from build123d import *

# Parameters (mm, degrees)
F0_W     = 1054.1
F0_H     = 781.05
F1_DEPTH = 304.8
F0_R     = 25.4
F2_DEPTH = 25.4
F3_R     = 12.7
F4_SIZE  = 3.175
F5_R     = 12.7


with BuildPart() as f1:
    # F0 (on Top) → F1 (new body)
    with BuildSketch(Plane.XY):
        Rectangle(F0_W, F0_H)
        with BuildLine():
            ThreePointArc((-24.260394, 317.953571), (-15.749117, 333.525595), (0.879086, 339.725))
            Line((0.879086, 339.725), (450.85, 339.725))
            ThreePointArc((450.85, 339.725), (468.810512, 332.285512), (476.25, 314.325))
            Line((476.25, 314.325), (476.25, -314.325))
            ThreePointArc((476.25, -314.325), (468.810512, -332.285512), (450.85, -339.725))
            Line((450.85, -339.725), (-450.85, -339.725))
            ThreePointArc((-450.85, -339.725), (-468.810512, -332.285512), (-476.25, -314.325))
            Line((-476.25, -314.325), (-476.25, -137.404086))
            ThreePointArc((-476.25, -137.404086), (-470.050595, -120.775883), (-454.478571, -112.264606))
            ThreePointArc((-454.478571, -112.264606), (-167.839755, 31.314755), (-24.260394, 317.953571))
        make_face(mode=Mode.SUBTRACT)
    extrude(amount=F1_DEPTH)

    # F0 (on Top) → F2 (join)
    with BuildSketch(Plane.XY):
        with BuildLine():
            Line((450.85, 339.725), (0.879086, 339.725))
            ThreePointArc((0.879086, 339.725), (-15.749117, 333.525595), (-24.260394, 317.953571))
            ThreePointArc((-24.260394, 317.953571), (-167.839755, 31.314755), (-454.478571, -112.264606))
            ThreePointArc((-454.478571, -112.264606), (-470.050595, -120.775883), (-476.25, -137.404086))
            Line((-476.25, -137.404086), (-476.25, -314.325))
            ThreePointArc((-476.25, -314.325), (-468.810512, -332.285512), (-450.85, -339.725))
            Line((-450.85, -339.725), (450.85, -339.725))
            ThreePointArc((450.85, -339.725), (468.810512, -332.285512), (476.25, -314.325))
            Line((476.25, -314.325), (476.25, 314.325))
            ThreePointArc((476.25, 314.325), (468.810512, 332.285512), (450.85, 339.725))
        make_face()
        with Locations((400.05, 0)):
            Circle(F0_R, mode=Mode.SUBTRACT)
    extrude(amount=F2_DEPTH)

    # F3
    f3_edges = [f1.edges().sort_by_distance(p)[0] for p in [
        (-167.839755, 31.314755, 304.8),
    ]]
    fillet(f3_edges, radius=F3_R)

    # F4
    f4_edges = [f1.edges().sort_by_distance(p)[0] for p in [
        (374.65, 0, 25.4),
    ]]
    chamfer(f4_edges, length=F4_SIZE)

    # F5
    f5_edges = [f1.edges().sort_by_distance(p)[0] for p in [
        (0, -390.525, 304.8),
    ]]
    fillet(f5_edges, radius=F5_R)


solid = f1.part
Design review of the part built by this model. Coordinates are the model's own, in mm. A direction names the side the tool comes from. Give positions to 0.01 mm unless a question says otherwise; leave off trailing zeros. Order: outer loops, then holes, each group sorted by start corner. A loop starts at its lowest first (then second) coordinate and runs counter-clockwise, first axis right, second up. Notation, with made-up numbers: (-7, 46) - (34, 46) arc R6 ccw to (34, 52) - close; hole circle Ø11 at (77.25, -0.75). An arc over 180 degrees is marked (long way). Write item = value, one per line. Start each with the question number.
Q1. We need section D-D on y = -253.5. State the section outline as (x, z) points.
Q2. Mouldability with a two-part tool opening along X and no side actions: class faces 3 (the face through (468.612, 332.482, 156.883)), 4 (the face through (-7, 390.525, 150)), 5 (the face through (-527.05, -5, 150)) as released by +X, released by -X, zero draft, split by the parting line, or undercut.
Q3. Tool access review of faces 1 (the face through (99, -71, 25.4)), 2 (the face through (374.675, 1.117, 10.957)): name each direction out of +Z, -Z, +X, -X, +Y, -Y from which nothing blocks a thin tool from reaching the whole face with its end or side.
Q4. To check wall thickness, follow L1, parallel to X at y = -260, z = 262.5; L2, parallel to Y at x = 400.05, z = 16 (3 decimals); L3, parallel to Y at x = 376.5, z = 242 (3 decimals). State the ranges of each line that lie inside material, in increasing order. Write a range as from..to.
Q5. We need section C-C on x = 256. State the section outline as (y, z) points (3 decimals).
Q6. We need section A-A on z = 112. State the section outline as (x, y) points (3 decimals).
Q7. We need section B-B on x = 400.05. State the section outline as (y, z) points (3 decimals), plus the area to 3 significant figures.
Working result:
q1.outline = (-527.05, 0) - (527.05, 0) - (527.05, 304.8) - (488.95, 304.8) arc R12.7 ccw to (476.25, 292.1) - (476.25, 25.4) - (-476.25, 25.4) - (-476.25, 292.1) arc R12.7 ccw to (-488.95, 304.8) - (-527.05, 304.8) - close
q2.face_3 = undercut
q2.face_4 = zero draft
q2.face_5 = released by -X
q3.face_1 = +Z
q3.face_2 = +Z, -Z
q4.L1 = -527.05..-476.25, 476.25..527.05
q4.L2 = -390.525..-25.4, 25.4..390.525
q4.L3 = -390.525..-339.725, 339.725..390.525
q5.outline = (-390.525, 0) - (390.525, 0) - (390.525, 304.8) - (352.425, 304.8) arc R12.7 ccw to (339.725, 292.1) - (339.725, 25.4) - (-339.725, 25.4) - (-339.725, 292.1) arc R12.7 ccw to (-352.425, 304.8) - (-377.825, 304.8) arc R12.7 ccw to (-390.525, 292.1) - close
q6.outline = (-527.05, -390.525) - (527.05, -390.525) - (527.05, 390.525) - (-527.05, 390.525) - close; hole (-476.25, -314.325) arc R25.4 ccw to (-450.85, -339.725) - (450.85, -339.725) arc R25.4 ccw to (476.25, -314.325) - (476.25, 314.325) arc R25.4 ccw to (450.85, 339.725) - (0.879, 339.725) arc R25.4 ccw to (-24.26, 317.954) arc R508 cw to (-454.479, -112.265) arc R25.4 ccw to (-476.25, -137.404) - close
q7.outline = (-390.525, 0) - (-25.4, 0) - (-25.4, 22.225) - (-28.575, 25.4) - (-339.725, 25.4) - (-339.725, 292.1) arc R12.7 ccw to (-352.425, 304.8) - (-377.825, 304.8) arc R12.7 ccw to (-390.525, 292.1) - close; (25.4, 0) - (390.525, 0) - (390.525, 304.8) - (352.425, 304.8) arc R12.7 ccw to (339.725, 292.1) - (339.725, 25.4) - (28.575, 25.4) - (25.4, 22.225) - close
q7.area = 46,800 mm²
